from build123d import *

# Parameters (mm, degrees)
SKETCH_2_R          = 35
SKETCH_2_R_2        = 5.5
EXTRUDE_1_DEPTH     = 5
EXTRUDE_START       = 15
SKETCH_3_R          = 35
SKETCH_3_R_2        = 30.1
EXTRUDE_2_DEPTH     = 15
SKETCH_4_R          = 1.55
CUT_EXTRUDE_1_DEPTH = 10
CUT_EXTRUDE_5_DEPTH = 15
FILLET_1_R          = 1
CUT_EXTRUDE_START   = -2
SKETCH_10_R         = 35
CUT_EXTRUDE_6_DEPTH = 2
CUT_EXTRUDE_7_DEPTH = 10
SKETCH1_R           = 9.130787709
CUT_EXTRUDE1_DEPTH  = 52.720402193


with BuildPart() as part:
    # 草图2 → 凸台-拉伸1 (new body)
    with BuildSketch(Plane.XY):
        Circle(SKETCH_2_R)
        Circle(SKETCH_2_R_2, mode=Mode.SUBTRACT)
    extrude(amount=EXTRUDE_1_DEPTH)

    # 草图3 → 凸台-拉伸2 (add)
    with BuildSketch(Plane(origin=(0, 0, 0), x_dir=(-1, 0, 0), z_dir=(0, 0, -1)).offset(EXTRUDE_START)):
        Circle(SKETCH_3_R)
        Circle(SKETCH_3_R_2, mode=Mode.SUBTRACT)
    extrude(amount=-EXTRUDE_2_DEPTH)

    # 草图4 → 切除-拉伸1 (cut)
    with BuildSketch(Plane(origin=(0, 0, -15), x_dir=(-1, 0, 0), z_dir=(0, 0, -1))):
        with Locations((0, 32.5)):
            Circle(SKETCH_4_R)
        with Locations((32.5, 0)):
            Circle(SKETCH_4_R)
        with Locations((0, -32.5)):
            Circle(SKETCH_4_R)
        with Locations((-32.5, 0)):
            Circle(SKETCH_4_R)
    extrude(amount=-CUT_EXTRUDE_1_DEPTH, mode=Mode.SUBTRACT)

    # 草图9 → 切除-拉伸5 (cut)
    with BuildSketch(Plane(origin=(0, 0, -15), x_dir=(-1, 0, 0), z_dir=(0, 0, -1))):
        with BuildLine():
            ThreePointArc((-22.013313369, 20.528615017), (-22.026376234, 22.026376234), (-20.528615017, 22.013313369))
            ThreePointArc((-20.528615017, 22.013313369), (-21.283914114, 21.283914114), (-22.013313369, 20.528615017))
        make_face()
        with BuildLine():
            ThreePointArc((20.528615017, 22.013313369), (22.026376234, 22.026376234), (22.013313369, 20.528615017))
            ThreePointArc((22.013313369, 20.528615017), (21.283914114, 21.283914114), (20.528615017, 22.013313369))
        make_face()
        with BuildLine():
            ThreePointArc((22.013313369, -20.528615017), (22.026376234, -22.026376234), (20.528615017, -22.013313369))
            ThreePointArc((20.528615017, -22.013313369), (21.283914114, -21.283914114), (22.013313369, -20.528615017))
        make_face()
        with BuildLine():
            ThreePointArc((-20.528615017, -22.013313369), (-22.026376234, -22.026376234), (-22.013313369, -20.528615017))
            ThreePointArc((-22.013313369, -20.528615017), (-21.283914114, -21.283914114), (-20.528615017, -22.013313369))
        make_face()
    extrude(amount=-CUT_EXTRUDE_5_DEPTH, mode=Mode.SUBTRACT)

    # 圆角1
    # the kernel refuses this fillet: 1 mm, written as the material it takes off along each edge
    with BuildSketch(Plane(origin=(0, 0, -15), x_dir=(-0.7403558797037455, 0.6722151228498904, 0), z_dir=(-0.6722151228498904, -0.7403558797037455, 0))) as fillet_1_piece_1:
        with BuildLine():
            CenterArc((30.1 + FILLET_1_R, -FILLET_1_R), FILLET_1_R, 90, 90)
            Line((30.1, -FILLET_1_R), (30.1, 0))
            Line((30.1, 0), (30.1 + FILLET_1_R, 0))
        make_face()
    revolve(axis=Axis((0, 0, -15), (0, 0, -1)), revolution_arc=95.523479776, mode=Mode.SUBTRACT)
    with BuildSketch(Plane(origin=(0, 0, -15), x_dir=(0.6722151228498918, 0.7403558797037441, 0), z_dir=(-0.7403558797037441, 0.6722151228498918, 0))) as fillet_1_piece_2:
        with BuildLine():
            CenterArc((30.1 + FILLET_1_R, -FILLET_1_R), FILLET_1_R, 90, 90)
            Line((30.1, -FILLET_1_R), (30.1, 0))
            Line((30.1, 0), (30.1 + FILLET_1_R, 0))
        make_face()
    revolve(axis=Axis((0, 0, -15), (0, 0, -1)), revolution_arc=95.523479776, mode=Mode.SUBTRACT)
    with BuildSketch(Plane(origin=(0, 0, -15), x_dir=(0.7403558797037453, -0.6722151228498905, 0), z_dir=(0.6722151228498905, 0.7403558797037453, 0))) as fillet_1_piece_3:
        with BuildLine():
            CenterArc((30.1 + FILLET_1_R, -FILLET_1_R), FILLET_1_R, 90, 90)
            Line((30.1, -FILLET_1_R), (30.1, 0))
            Line((30.1, 0), (30.1 + FILLET_1_R, 0))
        make_face()
    revolve(axis=Axis((0, 0, -15), (0, 0, -1)), revolution_arc=95.523479776, mode=Mode.SUBTRACT)
    with BuildSketch(Plane(origin=(0, 0, -15), x_dir=(-1, 0, 0), z_dir=(0, -1, 0))) as fillet_1_piece_4:
        with BuildLine():
            CenterArc((30.1 + FILLET_1_R, -FILLET_1_R), FILLET_1_R, 90, 90)
            Line((30.1, -FILLET_1_R), (30.1, 0))
            Line((30.1, 0), (30.1 + FILLET_1_R, 0))
        make_face()
    revolve(axis=Axis((0, 0, -15), (0, 0, -1)), revolution_arc=47.760430641, mode=Mode.SUBTRACT)
    with BuildSketch(Plane(origin=(0, 0, -15), x_dir=(-0.6722320403041436, -0.7403405189428228, 0), z_dir=(0.7403405189428228, -0.6722320403041436, 0))) as fillet_1_piece_5:
        with BuildLine():
            CenterArc((30.1 + FILLET_1_R, -FILLET_1_R), FILLET_1_R, 90, 90)
            Line((30.1, -FILLET_1_R), (30.1, 0))
            Line((30.1, 0), (30.1 + FILLET_1_R, 0))
        make_face()
    revolve(axis=Axis((0, 0, -15), (0, 0, -1)), revolution_arc=47.760430641, mode=Mode.SUBTRACT)

    # 草图10 → 切除-拉伸6 (cut)
    with BuildSketch(Plane.XY.offset(5).offset(CUT_EXTRUDE_START)):
        with Locations(Location((0, 0, 0), (0, 0, 180))):
            Circle(SKETCH_10_R)
    extrude(amount=CUT_EXTRUDE_6_DEPTH, mode=Mode.SUBTRACT)

    # 草图11 → 切除-拉伸7 (cut)
    with BuildSketch(Plane(origin=(0, 0, 0), x_dir=(-1, 0, 0), z_dir=(0, 0, -1))):
        with BuildLine():
            Line((12.990381057, 7.5), (15.588457268, 9))
            ThreePointArc((15.588457268, 9), (18, 0), (15.588457268, -9))
            Line((15.588457268, -9), (12.990381057, -7.5))
            ThreePointArc((12.990381057, -7.5), (15, 0), (12.990381057, 7.5))
        make_face()
        with BuildLine():
            Line((-7.5, 12.990381057), (-9, 15.588457268))
            ThreePointArc((-9, 15.588457268), (0, 18), (9, 15.588457268))
            Line((9, 15.588457268), (7.5, 12.990381057))
            ThreePointArc((7.5, 12.990381057), (0, 15), (-7.5, 12.990381057))
        make_face()
        with BuildLine():
            Line((7.5, -12.990381057), (9, -15.588457268))
            ThreePointArc((9, -15.588457268), (0, -18), (-9, -15.588457268))
            Line((-9, -15.588457268), (-7.5, -12.990381057))
            ThreePointArc((-7.5, -12.990381057), (0, -15), (7.5, -12.990381057))
        make_face()
        with BuildLine():
            Line((-12.990381057, -7.5), (-15.588457268, -9))
            ThreePointArc((-15.588457268, -9), (-18, 0), (-15.588457268, 9))
            Line((-15.588457268, 9), (-12.990381057, 7.5))
            ThreePointArc((-12.990381057, 7.5), (-15, 0), (-12.990381057, -7.5))
        make_face()
    extrude(amount=-CUT_EXTRUDE_7_DEPTH, mode=Mode.SUBTRACT)

    # Sketch1 → Cut-Extrude1 (cut, through all)
    with BuildSketch(Plane(origin=(0, 0, 0), x_dir=(-1, 0, 0), z_dir=(0, 0, -1))):
        Circle(SKETCH1_R)
    extrude(amount=-CUT_EXTRUDE1_DEPTH, mode=Mode.SUBTRACT)


solid = part.part
Design review of the part built by this model. Coordinates are the model's own, in mm. A direction names the side the tool comes from. Round coordinates to 2 decimals unless told otherwise and drop trailing zeros. Order: outer loops, then holes, each group sorted by start corner. A loop starts at its lowest first (then second) coordinate and runs counter-clockwise, first axis right, second up.
1) For L1, parallel to X at y = 0, z = -10; L2, parallel to Y at x = 0, z = 2.15, list the stretches that pass through material, from the lowest coordinate up.
The answers:
L1: x = -35 to -34.05, -30.95 to -30.1, 30.1 to 30.95, 34.05 to 35
L2: y = -35 to -18, -15 to -9.13, 9.13 to 15, 18 to 35
2) Machinability: for faces 4 (the cylindrical face through (0.202, 34.037, -10.07)), 5 (the flat face through (8.24, 14.27, 1.48)), which of the approach directions +Z, -Z, +X, -X, +Y, -Y give a long, thin tool a straight path to every point of the face, cutting with its end or side? Answer none if there is none.
The answers:
face 4: -Z
face 5: +Z, -Z
3) Consider section A-A (z = 1). State the section outline as (x, y) points.
The answers:
outline: circle Ø70 at (0, 0); hole (-15.59, -9) - (-12.99, -7.5) arc R15 cw to (-12.99, 7.5) - (-15.59, 9) arc R18 ccw to start; hole circle Ø18.26 at (0, 0); hole (-9, -15.59) arc R18 ccw to (9, -15.59) - (7.5, -12.99) arc R15 cw to (-7.5, -12.99) - close; hole (-9, 15.59) - (-7.5, 12.99) arc R15 cw to (7.5, 12.99) - (9, 15.59) arc R18 ccw to start; hole (12.99, -7.5) - (15.59, -9) arc R18 ccw to (15.59, 9) - (12.99, 7.5) arc R15 cw to start
4) Draft analysis for pull direction Y (two halves, no side actions). For faces 1 (the flat face through (-7, 7, 3)), 2 (the cylindrical face through (-22.04, -22.01, -7.6)), 3 (the flat face through (0, -32, -5)), state which applies: released by +Y, released by -Y, zero draft, split by the parting line, or undercut.
The answers:
face 1: zero draft
face 2: undercut
face 3: undercut
5) Clearance check with flat-ended pins moving along their axes: pin 1 Ø8 at (y, z) = (-24.5, -8.5) entering from +X; pin 2 Ø0.5 at (x, y) = (21.5, -21) entering from -Z; pin 3 Ø1.5 at (x, y) = (0, 32.5) entering from -Z; pin 4 Ø1.5 at (x, y) = (-33, 1) entering from -Z. State where each tip first meets the part, or that it passes through.
The answers:
pin 1: stops at x = 28.37
pin 2: stops at z = 0
pin 3: stops at z = -5
pin 4: stops at z = -15
6) Consider section B-B (x = -32.5). State the section outline as (y, z) points, plus the area to 3 significant figures.
The answers:
outline: (-12.99, -15) - (-1.55, -15) - (-1.55, -5) - (1.55, -5) - (1.55, -15) - (12.99, -15) - (12.99, 3) - (-12.99, 3) - close
area: 437 mm2
7) Consider section D-D (y = -3). Count the separate pieces of the cut face and the enclosed holes in it, plus the area to 3 significant figures.
The answers:
separate pieces: 4
enclosed holes: 0
area: 286 mm2
